Check sheet for the drawn part. Datum: minimum x, y, z corner. Units: mm. Give positions to 0.01 mm unless a question says otherwise; leave off trailing zeros. Write each loop counter-clockwise with the first axis right and the second up, starting at its lowest first coordinate (ties: lowest second). Pieces come first, ordered by that corner, then holes.
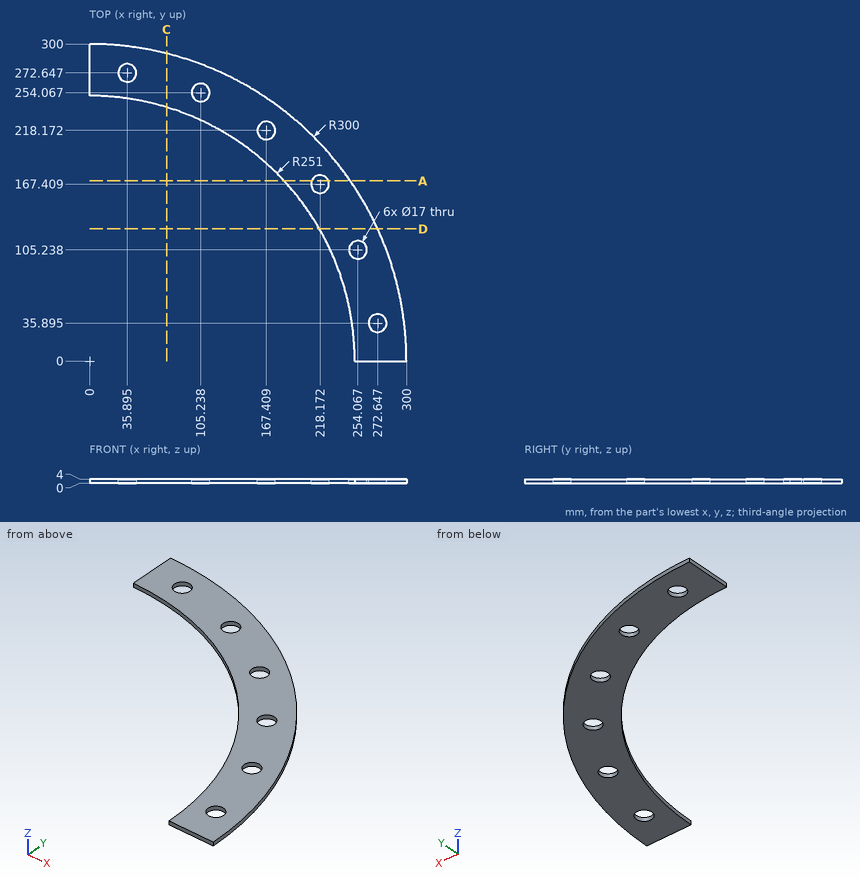
1) Sectioned sample at A-A on y = 170.5. Record the boundary of the cut face in (x, z), then the cut area to 3 significant figures.
2) Sectioned sample at D-D on y = 125. Record the boundary of the cut face in (x, z), then the cut area to 3 significant figures.
3) Sectioned sample at C-C on x = 73. Record the boundary of the cut face in (y, z), then the cut area to 3 significant figures.
4) Gauge pin test, flat ends, axial feed: pin 1 (1 mm diameter, centred on x = 155, z = 1, fed in from +Y); pin 2 (2 mm diameter, centred on x = 72, z = 0.5, fed in from -Y); pin 3 (2 mm diameter, centred on y = 100, z = 3, fed in from +X) (1 decimal). Record the tip position at first contact, or that the pin passes through.
5) Scan lines: L1, parallel to Y at x = 168.5, z = 0.35 (1 decimal); L2, parallel to Y at x = 218, z = 2.45 (1 decimal); L3, parallel to X at y = 223.5, z = 1.5 (1 decimal). Record each from-to range of solid material in increasing order.
Answers below:
1. outline: (184.2, 0) - (210.25, 0) - (210.25, 4) - (184.2, 4) - close; (226.09, 0) - (246.84, 0) - (246.84, 4) - (226.09, 4) - close
1. area: 187 mm2
2. outline: (217.66, 0) - (272.72, 0) - (272.72, 4) - (217.66, 4) - close
2. area: 220 mm2
3. outline: (240.15, 0) - (290.98, 0) - (290.98, 4) - (240.15, 4) - close
3. area: 203 mm2
4. pin 1: stops at y = 257.16
4. pin 2: stops at y = 240.15
4. pin 3: stops at x = 283.2
5. L1: y = 186 to 209.7, 226.6 to 248.2
5. L2: y = 124.4 to 158.9, 175.9 to 206.1
5. L3: x = 114.2 to 160.8, 174 to 200.1
